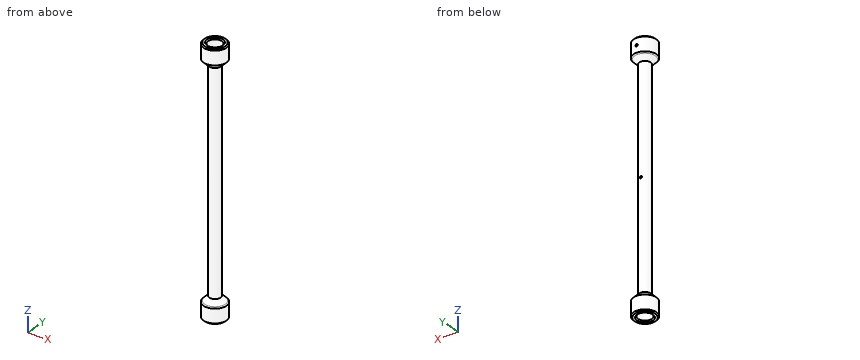
Autodesk Inventor part; units mm, degrees
ref_plane "Work Plane1" through (0, 5, -3.5) normal (0, 1, 0) x (-1, 0, 0)
ref_plane "Work Plane2" through (0, 2.5, -56) normal (0, 1, 0) x (-1, 0, 0)
ref_plane "YZ Plane" through (0, 0, 0) normal (1, 0, 0) x (0, 1, 0)
sketch "Sketch1" plane through (0, 0, 0) normal (1, 0, 0) x (0, 1, 0)
  line L0 (0, 0) -> (0, -112)
  line L1 (0, -112) -> (3, -112)
  line L2 (3, -112) -> (3, 0)
  line L3 (3, 0) -> (0, 0)
  line L4 (3, 0) -> (3, -6)
  line L5 (3, -112) -> (3, -106)
  line L6 (3, -112) -> (5, -112)
  line L7 (5, -112) -> (5, -106)
  line L8 (5, -106) -> (3, -106)
  line L9 (3, 0) -> (5, 0)
  line L10 (5, 0) -> (5, -6)
  line L11 (5, -6) -> (3, -6)
  line L12 (3, -106) -> (0.5, -106)
  line L13 (0.5, -106) -> (0.5, -6)
  line L14 (0.5, -6) -> (3, -6)
  line L15 (5, -6) -> (5, -7)
  line L16 (5, -7) -> (0.5, -7)
  line L17 (5, -106) -> (5, -105)
  line L18 (5, -105) -> (0.5, -105)
  line L19 (3, -7) -> (3.1, -7)
  line L20 (2.5, -7) -> (2.5, -105)
  point P0 (3, -105)
  point P1 (2, -6)
  point P2 (3.1, -105)
  dimension "d0" = 112
  dimension "d1" = 3
  dimension "d2" = 6
  dimension "d3" = 6
  dimension "d5" = 2
  dimension "d6" = 2
  dimension "d7" = 2.5
  dimension "d8" = 1
  dimension "d9" = 1
  dimension "d22" = 2
revolve "Revolution1" add sketch "Sketch1" angle 360 about axis through (0, 0, 0) along (0, 0, -1) contours L9 L10 L11 L2 | L2 L8 L7 L6 | L11 L15 L16 L2 | L2 L16 L13 L14 | L12 L13 L18 L2 | L2 L18 L17 L8 | L20 L18 L13 L16
thread "Thread1"
thread "Thread2"
chamfer "Chamfer1" distance 0.5 angle 45 2 edges at (0, -3, 0) (0, -3, -112)
chamfer "Chamfer2" distance 0.5 angle 45 4 edges at (0, -5, -112) (0, -5, -105) (0, -5, -7) (0, -5, 0)
chamfer "Chamfer3" distance 2 angle 45 2 edges at (0, -2.5, -7) (0, -2.5, -105)
ref_plane "Work Plane1" through (0, 5, -3.5) normal (0, 1, 0) x (-1, 0, 0)
ref_plane "Work Plane2" through (0, 2.5, -56) normal (0, 1, 0) x (-1, 0, 0)
sketch "Sketch2" plane through (0, 5, -3.5) normal (0, 1, 0) x (-1, 0, 0)
  point P0 (0, 3.5)
  point P1 (0, 0)
  point P2 (0, 0)
sketch "Sketch3" plane through (0, 2.5, -56) normal (0, 1, 0) x (-1, 0, 0)
  point P0 (0, 56)
  point P1 (0, 0)
hole "Hole1" at (0, 5, -3.5) direction (0, -1, 0) diameter 1 depth 0.5 tip angle 118
hole "Hole2" at (0, 2.5, -56) direction (0, -1, 0) diameter 1 depth 0.5 tip angle 118
properties part number "Heater"
Could you check a few things on this model? Use its own coordinates, in mm. Give positions to 0.01 mm unless a question says otherwise; leave off trailing zeros. Write each loop counter-clockwise with the first axis right and the second up, starting at its lowest first coordinate (ties: lowest second). Pieces come first, ordered by that corner, then holes. Notation, with made-up numbers: (70.5, -32) - (88.5, -32) arc R10 cw to (88.5, -21) - close; hole circle Ø10 at (72, 75). An arc over 180 degrees is marked (long way). Use CSV: the item, a comma, the result in double quotes. Start each with the question number.
Item 1: I'm going to push flat-ended pins straight in: pin 1 (5 mm diameter, centred on x = 0, y = 0, fed in from +Z); pin 2 (4 mm diameter, centred on x = 0, z = -43, fed in from +Y); pin 3 (4 mm diameter, centred on y = -2.5, z = -29.5, fed in from -X). Where does each tip first touch, or does it pass through?
Item 2: If I drill on line 1 along Z through (x, y) = (0, 2.35); line 2 along Z through (x, y) = (-3.75, 2.5); line 3 along X through (y, z) = (0, -31.5), over which ranges is the centre line in solid material (lowest first)?
Item 3: I want a section at A-A, the plane z = -97.5. Please give me the cut outline in (x, y).
Findings:
1,pin 1,"stops at z = -6"
1,pin 2,"stops at y = 2.5"
1,pin 3,"stops at x = -2.45"
2,line 1,"z = -106 to -56.5, -55.5 to -6"
2,line 2,"z = -111.99 to -105.01, -6.99 to -0.01"
2,line 3,"x = -2.5 to -0.5, 0.5 to 2.5"
3,outline,"circle Ø5 at (0, 0); hole circle Ø1 at (0, 0)"
